Read the model definition and answer for the solid it produces. Units are mm, in the model's axes. A direction names the side the tool comes from. Round coordinates to 2 decimals unless told otherwise and drop trailing zeros. Loops run counter-clockwise (first coordinate to the right, second up) from the corner with the lowest first, then second, coordinate; pieces in that order, holes last. Notation, with made-up numbers: M 4.25,36.5 L 49.25,36.5 A33 ccw 49.25,70.5 Z; hole C 8,18.25 d8. An arc over 180 degrees is marked long. Write each question's results on one line, items separated by ' | '.
```python
from build123d import *

# Parameters (mm, degrees)
F1_DEPTH             = 20
F4_D                 = 3.3
F4_CSINK_D           = 6.72
F4_CSINK_ANGLE       = 90
F4_ON_F2_D           = 3.3
F4_ON_F2_CSINK_D     = 6.72
F4_ON_F2_CSINK_ANGLE = 90
F5_SIZE              = 1


with BuildPart() as f1:
    # F0 (on Front) → F1 (new body)
    with BuildSketch(Plane.XZ):
        Polygon((0, 2), (0, 0), (12, 0), (12, 9.7012996929), (22, 9.7012996929), (22, 0), (34, 0), (34, 2), (24, 2), (24, 11.7012996929), (10, 11.7012996929), (10, 2), align=None)
    extrude(amount=F1_DEPTH)

    # F4 (through all)
    with Locations(Plane.XY.offset(2)):
        with Locations((5, -10)):
            CounterSinkHole(F4_D / 2, F4_CSINK_D / 2, counter_sink_angle=F4_CSINK_ANGLE)

    # F4 on F2 (through all)
    with Locations(Plane.XY.offset(2)):
        with Locations((29, -10)):
            CounterSinkHole(F4_ON_F2_D / 2, F4_ON_F2_CSINK_D / 2, counter_sink_angle=F4_ON_F2_CSINK_ANGLE)

    # F5
    f5_edges = [f1.edges().sort_by_distance(p)[0] for p in [
        (24, -10, 2),
        (10, -10, 2),
    ]]
    chamfer(f5_edges, length=F5_SIZE)


solid = f1.part
```
1. Given P1, Ø8, axis at x = 28.5, y = -4.5, coming from the +Z side; P2, Ø2.5, axis at x = 5.5, y = -12, coming from the +Z side; P3, Ø3, axis at x = 5, y = -10, coming from the -Z side; P4, Ø3, axis at y = -13.5, z = 7, coming from the -X side, each flat-ended and moving along its own axis, determine where each tip first touches the part or whether it passes through.
Completed:
P1: stops at z = 2.5 | P2: stops at z = 1.95 | P3: passes through | P4: stops at x = 10
2. Which of the six approach directions +Z, -Z, +X, -X, +Y, -Y give full straight-line access (tool end or side, diameter ignored) to faces 4 (the face through (7, -10, 0)), 5 (the face through (32, -8, 2)), 6 (the face through (17, -10, 9.701)), 7 (the face through (10, -10, 7))?
Completed:
face 4: -Z, +X, -X, +Y, -Y | face 5: +Z, +X, +Y, -Y | face 6: -Z, +Y, -Y | face 7: +Z, -X, +Y, -Y
3. Determine the mould class of faces 1 (the face through (9.5, -9.9, 2.5)), 2 (the face through (24, -10, 7)), 3 (the face through (22, -10, 5)) for opening direction X: released by +X, released by -X, zero draft, split by the parting line, or undercut.
Completed:
face 1: released by -X | face 2: released by +X | face 3: undercut
4. Find section C-C, the plane z = 3.75. Give the vertices of the cut face in (x, y), then the cut area to 3 significant figures.
Completed:
outline: M 10,-20 L 12,-20 L 12,0 L 10,0 Z; M 22,-20 L 24,-20 L 24,0 L 22,0 Z | area: 80.0 mm2
5. Find the intervals of material crossed by L1, parallel to X at y = -10, z = 0.25; L2, parallel to X at y = -1.75, z = 1.75; L3, parallel to X at y = -10, z = 5, in increasing order.
Completed:
L1: x = 0 to 3.35, 6.65 to 12, 22 to 27.35, 30.65 to 34 | L2: x = 0 to 12, 22 to 34 | L3: x = 10 to 12, 22 to 24
6. Find section B-B, the plane y = -10. Give the vertices of the cut face in (x, z).
Completed:
outline: M 0,0 L 3.35,0 L 3.35,0.29 L 1.64,2 L 0,2 Z; M 6.65,0 L 12,0 L 12,9.7 L 22,9.7 L 22,0 L 27.35,0 L 27.35,0.29 L 25.64,2 L 25,2 L 24,3 L 24,11.7 L 10,11.7 L 10,3 L 9,2 L 8.36,2 L 6.65,0.29 Z; M 30.65,0 L 34,0 L 34,2 L 32.36,2 L 30.65,0.29 Z
7. Find section D-D, the plane x = 5. Give the vertices of the cut face in (y, z), then the cut area to 3 significant figures.
Completed:
outline: M -20,0 L -11.65,0 L -11.65,0.29 L -13.36,2 L -20,2 Z; M -8.35,0 L 0,0 L 0,2 L -6.64,2 L -8.35,0.29 Z | area: 30.5 mm2
8. Find section A-A, the plane z = 1. Give the vertices of the cut face in (x, y).
Completed:
outline: M 0,-20 L 12,-20 L 12,0 L 0,0 Z; M 22,-20 L 34,-20 L 34,0 L 22,0 Z; hole C 5,-10 d4.72; hole C 29,-10 d4.72
